```python
from build123d import *

# Parameters (mm, degrees)
SKETCH1_W                                       = 50.8
SKETCH1_H                                       = 88.9
BOSS_EXTRUDE1_DEPTH                             = 12.7
CSK_FOR_M4_FLAT_HEAD_MACHINE_SCREW1_D           = 4.5
CSK_FOR_M4_FLAT_HEAD_MACHINE_SCREW1_CSINK_D     = 9.4
CSK_FOR_M4_FLAT_HEAD_MACHINE_SCREW1_CSINK_ANGLE = 90
CBORE_FOR_10_SOCKET_HEAD_CAP_SCREW1_D           = 5.1054
CBORE_FOR_10_SOCKET_HEAD_CAP_SCREW1_CBORE_D     = 9.525
CBORE_FOR_10_SOCKET_HEAD_CAP_SCREW1_CBORE_DEPTH = 4.826


with BuildPart() as part:
    # Sketch1 → Boss-Extrude1 (new body)
    with BuildSketch(Plane(origin=(0, 0, 0), x_dir=(0, 0, -1), z_dir=(1, 0, 0))):
        Rectangle(SKETCH1_W, SKETCH1_H)
    extrude(amount=BOSS_EXTRUDE1_DEPTH)

    # CSK for M4 Flat Head Machine Screw1 (through all)
    with Locations(Plane(origin=(12.7, 0, 0), x_dir=(0, 0, -1), z_dir=(1, 0, 0))):
        with Locations((11.136931804, 34.973863607), (-11.136931804, 34.973863607), (-11.136931804, 12.7), (11.136931804, 12.7)):
            CounterSinkHole(CSK_FOR_M4_FLAT_HEAD_MACHINE_SCREW1_D / 2, CSK_FOR_M4_FLAT_HEAD_MACHINE_SCREW1_CSINK_D / 2, counter_sink_angle=CSK_FOR_M4_FLAT_HEAD_MACHINE_SCREW1_CSINK_ANGLE)

    # CBORE for #10 Socket Head Cap Screw1 (through all)
    with Locations(Plane.ZY):
        with Locations((-15.875, -31.75), (0, -31.75), (15.875, -31.75)):
            CounterBoreHole(CBORE_FOR_10_SOCKET_HEAD_CAP_SCREW1_D / 2, CBORE_FOR_10_SOCKET_HEAD_CAP_SCREW1_CBORE_D / 2, CBORE_FOR_10_SOCKET_HEAD_CAP_SCREW1_CBORE_DEPTH)


solid = part.part
```
Check sheet for the modelled part. Datum: model origin and axes. Units: mm. A direction names the side the tool comes from. Coordinates: 2 decimals unless noted, no trailing zeros. Order: outer loops, then holes, each group sorted by start corner. A loop starts at its lowest first (then second) coordinate and runs counter-clockwise, first axis right, second up. Notation, with made-up numbers: M 35,48.5 L 61,48.5 A26 ccw 61,79.5 Z; hole C 22,47 d1. An arc over 180 degrees is marked long. One line per question, with ' | ' between items. Start each with the question number.
Item 1: Sectioned sample at D-D on x = 4. Count the separate pieces of the cut face and the enclosed holes in it, and give its area (3 significant figures).
Item 2: Material ranges on line 1 (Z direction, x = 4.75, y = 12.7); line 2 (Y direction, x = 7.75, z = -13); line 3 (Y direction, x = 12, z = -14), recorded low to high.
Item 3: Sectioned sample at C-C on y = -31.75. Record the cut outline in (x, z), and give its area (3 significant figures).
Item 4: Gauge pin test, flat ends, axial feed: P1, Ø8.5, axis at y = -31.75, z = 15.875, coming from the -X side; P2, Ø5, axis at y = 12.7, z = 11.14, coming from the +X side; P3, Ø6, axis at y = 12.7, z = -11.14, coming from the +X side. Record the tip position at first contact, or that the pin passes through.
Item 5: Access from +Z, -Z, +X, -X, +Y, -Y to the whole of each face (thin tool, end or side, straight path). Record for faces 1 (the flat face through (4.826, -34, -14)), 2 (the cylindrical face through (5.053, 32.978, -10.099)).
Item 6: Mould release check, pull along Y, two halves, no side actions. Record for faces 3 (the flat face through (6, -44.45, 0)), 4 (the cylindrical face through (8.818, -34.242, 0.553)), 5 (the flat face through (12.7, 1, 0)): pulls with the +Y half, pulls with the -Y half, needs draft (parallel to the pull), parting line crosses it, or undercut.
Item 7: Sectioned sample at A-A on y = 12.7. Record the cut outline in (x, z), and give its area (3 significant figures).
Item 8: Sectioned sample at B-B on z = 0. Record the cut outline in (x, y).
Answer below:
1) separate pieces: 1 | enclosed holes: 7 | area: 4,240 mm^2
2) line 1: z = -25.4 to -13.39, -8.89 to 8.89, 13.39 to 25.4 | line 2: y = -44.45 to 11.44, 13.96 to 33.71, 36.24 to 44.45 | line 3: y = -44.45 to -33.48, -30.02 to 9.91, 15.49 to 32.18, 37.77 to 44.45
3) outline: M 0,-25.4 L 12.7,-25.4 L 12.7,-18.43 L 4.83,-18.43 L 4.83,-20.64 L 0,-20.64 Z; M 0,-11.11 L 4.83,-11.11 L 4.83,-13.32 L 12.7,-13.32 L 12.7,-2.55 L 4.83,-2.55 L 4.83,-4.76 L 0,-4.76 Z; M 0,4.76 L 4.83,4.76 L 4.83,2.55 L 12.7,2.55 L 12.7,13.32 L 4.83,13.32 L 4.83,11.11 L 0,11.11 Z; M 0,20.64 L 4.83,20.64 L 4.83,18.43 L 12.7,18.43 L 12.7,25.4 L 0,25.4 Z | area: 387 mm^2
4) P1: stops at x = 4.83 | P2: stops at x = 10.5 | P3: stops at x = 11
5) face 1: -X | face 2: +X, -X
6) face 3: pulls with the -Y half | face 4: undercut | face 5: needs draft
7) outline: M 0,-25.4 L 12.7,-25.4 L 12.7,-15.84 L 10.25,-13.39 L 0,-13.39 Z; M 0,-8.89 L 10.25,-8.89 L 12.7,-6.44 L 12.7,6.44 L 10.25,8.89 L 0,8.89 Z; M 0,13.39 L 10.25,13.39 L 12.7,15.84 L 12.7,25.4 L 0,25.4 Z | area: 519 mm^2
8) outline: M 0,-44.45 L 12.7,-44.45 L 12.7,-34.3 L 4.83,-34.3 L 4.83,-36.51 L 0,-36.51 Z; M 0,-26.99 L 4.83,-26.99 L 4.83,-29.2 L 12.7,-29.2 L 12.7,44.45 L 0,44.45 Z
